from build123d import *

# Parameters (mm, degrees)
SKETCH1_W           = 78
SKETCH1_H           = 60
BOSS_EXTRUDE1_DEPTH = 5
SKETCH2_W           = 34
SKETCH2_H           = 40
BOSS_EXTRUDE2_DEPTH = 15
SKETCH4_W           = 7
SKETCH4_H           = 10
CUT_EXTRUDE1_DEPTH  = 15
SKETCH5_W           = 14
SKETCH5_H           = 11
CUT_EXTRUDE2_DEPTH  = 67.615484892
SKETCH6_W           = 11
SKETCH6_H           = 14
CUT_EXTRUDE3_DEPTH  = 72.170921878
SKETCH7_R           = 3
CUT_EXTRUDE4_DEPTH  = 58.375281685


with BuildPart() as part:
    # Sketch1 → Boss-Extrude1 (new body)
    with BuildSketch(Plane.XY):
        with Locations((-0.21253406, 9.10626703)):
            Rectangle(SKETCH1_W, SKETCH1_H)
    extrude(amount=BOSS_EXTRUDE1_DEPTH)

    # Sketch2 → Boss-Extrude2 (add)
    with BuildSketch(Plane.XY.offset(5)):
        with Locations((-0.21253406, 9.10626703)):
            Rectangle(SKETCH2_W, SKETCH2_H)
    extrude(amount=BOSS_EXTRUDE2_DEPTH)

    # Sketch4 → Cut-Extrude1 (cut)
    with BuildSketch(Plane.XY.offset(20)):
        with Locations((-13.71253406, 24.10626703)):
            Rectangle(SKETCH4_W, SKETCH4_H)
        with Locations((13.28746594, 24.10626703)):
            Rectangle(SKETCH4_W, SKETCH4_H)
        with Locations((13.28746594, -5.89373297)):
            Rectangle(SKETCH4_W, SKETCH4_H)
        with Locations((-13.71253406, -5.89373297)):
            Rectangle(SKETCH4_W, SKETCH4_H)
    extrude(amount=-CUT_EXTRUDE1_DEPTH, mode=Mode.SUBTRACT)

    # Sketch5 → Cut-Extrude2 (cut, through all)
    with BuildSketch(Plane.XZ.offset(10.89373297)):
        with Locations((-0.21253406, 12.5)):
            Rectangle(SKETCH5_W, SKETCH5_H)
    extrude(amount=-CUT_EXTRUDE2_DEPTH, mode=Mode.SUBTRACT)

    # Sketch6 → Cut-Extrude3 (cut, through all)
    with BuildSketch(Plane(origin=(16.78746594, 0, 0), x_dir=(0, 0, -1), z_dir=(1, 0, 0))):
        with Locations((-12.5, 9.10626703)):
            Rectangle(SKETCH6_W, SKETCH6_H)
    extrude(amount=-CUT_EXTRUDE3_DEPTH, mode=Mode.SUBTRACT)

    # Sketch7 → Cut-Extrude4 (cut, through all)
    with BuildSketch(Plane.XY.offset(5)):
        with Locations((-23.21253406, 24.10626703)):
            Circle(SKETCH7_R)
        with Locations((22.78746594, 24.10626703)):
            Circle(SKETCH7_R)
        with Locations((22.78746594, -5.89373297)):
            Circle(SKETCH7_R)
        with Locations((-23.21253406, -5.89373297)):
            Circle(SKETCH7_R)
    extrude(amount=-CUT_EXTRUDE4_DEPTH, mode=Mode.SUBTRACT)


solid = part.part
The listing builds one solid part. Answer for the finished solid, in the listing's coordinates (mm). A direction names the side the tool comes from. Give positions to 0.01 mm unless a question says otherwise; leave off trailing zeros. Loops run counter-clockwise (first coordinate to the right, second up) from the corner with the lowest first, then second, coordinate; pieces in that order, holes last. Notation, with made-up numbers: M 41,40 L 85,40 A20 cw 85,46 Z; hole C 28,51 d2. An arc over 180 degrees is marked long. Answer as CSV lines item,"result".
Item 1: The part is cut by section D-D (x = 8). Give the vertices of the cut face in (y, z), and give its area (3 significant figures).
Values follow:
outline,"M -20.89,0 L 39.11,0 L 39.11,5 L 29.11,5 L 29.11,20 L -10.89,20 L -10.89,5 L -20.89,5 Z; hole M 2.11,7 L 16.11,7 L 16.11,18 L 2.11,18 Z"
area,"746 mm^2"
Item 2: The mould has two halves that part along Z. Classify faces 5 (the flat face through (13, 19.106, 13)), 6 (the flat face through (-7.213, 23, 12)): released by +Z, released by -Z, zero draft, split by the parting line, or undercut.
Values follow:
face 5,"zero draft"
face 6,"undercut"
Item 3: Given pin 1 Ø8 at (x, z) = (-21, 17.5) entering from +Y; pin 2 Ø5 at (y, z) = (23.5, 15.5) entering from -X; pin 3 Ø3 at (y, z) = (-0.5, 12.5) entering from +X; pin 4 Ø5 at (x, y) = (-23.21, 24.11) entering from -Z, each flat-ended and moving along its own axis, determine where each tip first touches the part or whether it passes through.
Values follow:
pin 1,"stops at y = 19.11"
pin 2,"stops at x = -10.21"
pin 3,"stops at x = 16.79"
pin 4,"passes through"
Item 4: The part is cut by section C-C (x = -23). Give the vertices of the cut face in (y, z).
Values follow:
outline,"M -20.89,0 L -8.89,0 L -8.89,5 L -20.89,5 Z; M -2.9,0 L 21.11,0 L 21.11,5 L -2.9,5 Z; M 27.1,0 L 39.11,0 L 39.11,5 L 27.1,5 Z"
Item 5: The part is cut by section A-A (z = 12.75). Give the vertices of the cut face in (x, y).
Values follow:
outline,"M -17.21,-0.89 L -10.21,-0.89 L -10.21,-10.89 L -7.21,-10.89 L -7.21,2.11 L -17.21,2.11 Z; M -17.21,16.11 L -7.21,16.11 L -7.21,29.11 L -10.21,29.11 L -10.21,19.11 L -17.21,19.11 Z; M 6.79,-10.89 L 9.79,-10.89 L 9.79,-0.89 L 16.79,-0.89 L 16.79,2.11 L 6.79,2.11 Z; M 6.79,16.11 L 16.79,16.11 L 16.79,19.11 L 9.79,19.11 L 9.79,29.11 L 6.79,29.11 Z"
Item 6: Which of the six approach directions +Z, -Z, +X, -X, +Y, -Y give full straight-line access (tool end or side, diameter ignored) to faces 1 (the flat face through (-12, 2.106, 13)), 2 (the flat face through (0, 9, 18)), 3 (the flat face through (-10.213, 24, 13)), 4 (the flat face through (0, -10.894, 19))?
Values follow:
face 1,"+X, -X"
face 2,"none"
face 3,"+Z, -X, +Y"
face 4,"+Z, +X, -X, -Y"
Item 7: The part is cut by section B-B (y = 5). Give the vertices of the cut face in (x, z).
Values follow:
outline,"M -39.21,0 L 38.79,0 L 38.79,5 L 16.79,5 L 16.79,7 L -17.21,7 L -17.21,5 L -39.21,5 Z; M -17.21,18 L 16.79,18 L 16.79,20 L -17.21,20 Z"
Item 8: Straight lines are drawn through the part: line 1 along X through (y, z) = (1, 10); line 2 along X through (y, z) = (-10, 15.25); line 3 along Z through (x, y) = (4, -10.5). For each, find the intervals that lie inside material, in ascending order. Write a range as [from, to].
Values follow:
line 1,"x = [-17.21, -7.21], [6.79, 16.79]"
line 2,"x = [-10.21, -7.21], [6.79, 9.79]"
line 3,"z = [0, 7], [18, 20]"
